Autodesk Inventor part; units mm, degrees
ref_plane "YZ Plane" through (0, 0, 0) normal (1, 0, 0) x (0, 1, 0)
ref_plane "XZ Plane" through (0, 0, 0) normal (0, 1, 0) x (-1, 0, 0)
ref_plane "XY Plane" through (0, 0, 0) normal (0, 0, 1) x (1, 0, 0)
sketch "Sketch1" plane through (0, 0, 0) normal (0, 0, 1) x (1, 0, 0)
  line L0 (10.2242, -22.1045) -> (46.869, -22.1045) construction
  line L1 (46.869, -22.1045) -> (46.869, -51.7203) construction
  line L2 (46.869, -51.7203) -> (10.2242, -51.7203) construction
  line L3 (10.2242, -51.7203) -> (10.2242, -22.1045) construction
  line L4 (29.8676, -31.4438) -> (29.8676, -43.4438) construction
  line L5 (33.8496, -35.029) -> (33.8496, -42.667)
  line L6 (33.8496, -42.667) -> (33.8496, -43.4438)
  line L7 (33.8496, -43.4438) -> (32.8496, -43.4438)
  line L8 (22.8496, -43.4438) -> (22.8496, -42.4438)
  line L9 (22.8496, -31.4438) -> (25.8496, -31.4438)
  line L10 (33.8496, -31.4438) -> (33.8496, -35.019)
  line L11 (28.3496, -31.4438) -> (28.3496, -43.4438) construction
  line L12 (28.3496, -31.4438) -> (25.8496, -31.4438)
  line L13 (25.8496, -31.4438) -> (22.8496, -35.019)
  line L14 (28.3496, -43.4438) -> (23.8496, -43.4438)
  line L15 (23.8496, -43.4438) -> (22.8496, -42.4438)
  line L16 (30.8496, -31.4438) -> (33.8496, -35.019)
  line L17 (32.8496, -43.4438) -> (33.8496, -42.4438)
  line L18 (25.8496, -31.4438) -> (30.8496, -31.4438)
  line L19 (22.8496, -35.019) -> (22.8496, -31.4438)
  line L20 (23.8496, -43.4438) -> (22.8496, -43.4438)
  line L21 (22.8496, -42.4438) -> (22.8496, -35.019)
  line L22 (32.8496, -43.4438) -> (23.8496, -43.4438)
  line L23 (33.8496, -43.4438) -> (33.8496, -43.6998)
  line L24 (33.8496, -42.4438) -> (33.8496, -43.4438)
  line L25 (33.8496, -35.019) -> (33.8496, -42.4438)
  line L26 (30.8496, -31.4438) -> (33.8496, -31.4438)
  circle A0 centre (28.3496, -36.9438) radius 2
  line L27 (26.6175, -35.9438) -> (30.0816, -35.9438)
  line L28 (25.0671, -43.4438) -> (25.3808, -43.8918)
  line L29 (25.0671, -43.4438) -> (25.614, -43.4438) construction
  line L30 (25.3808, -43.8918) -> (25.3808, -45.1736)
  line L31 (25.3808, -45.1736) -> (26.2783, -45.1736)
  line L32 (26.2783, -45.1736) -> (26.2783, -43.9789)
  line L33 (26.2783, -43.9789) -> (26.5414, -43.4438)
  line L34 (27.5656, -43.4438) -> (27.8793, -43.8918)
  line L35 (27.8793, -43.8918) -> (27.8793, -45.1736)
  line L36 (27.8793, -45.1736) -> (28.7769, -45.1736)
  line L37 (28.7769, -45.1736) -> (28.7769, -43.9789)
  line L38 (28.7769, -43.9789) -> (29.04, -43.4438)
  line L39 (31.6321, -43.4438) -> (31.3184, -43.8918)
  line L40 (31.3184, -43.8918) -> (31.3184, -45.1736)
  line L41 (31.3184, -45.1736) -> (30.4209, -45.1736)
  line L42 (30.4209, -45.1736) -> (30.4209, -43.9789)
  line L43 (30.4209, -43.9789) -> (30.1577, -43.4438)
  line L44 (31.6321, -43.4438) -> (31.3184, -43.8918)
  line L45 (31.3184, -43.8918) -> (31.3184, -45.1736)
  line L46 (31.3184, -45.1736) -> (30.4209, -45.1736)
  line L47 (30.4209, -45.1736) -> (30.4209, -43.9789)
  line L48 (30.4209, -43.9789) -> (30.1577, -43.4438)
  line L49 (31.6321, -43.4438) -> (31.3184, -43.8918)
  line L50 (31.3184, -43.8918) -> (31.3184, -45.1736)
  line L51 (31.3184, -45.1736) -> (30.4209, -45.1736)
  line L52 (30.4209, -45.1736) -> (30.4209, -43.9789)
  line L53 (30.4209, -43.9789) -> (30.1577, -43.4438)
  line L54 (28.7769, -30.3247) -> (27.8793, -30.3247)
  line L55 (27.8793, -30.3247) -> (27.8793, -31.4438)
  line L56 (27.8793, -31.4438) -> (28.7769, -31.4438)
  line L57 (28.7769, -31.4438) -> (28.7769, -30.3247)
  point P0 (0, 0)
  dimension "d1" = 12
  dimension "d57" = 11
  dimension "d58" = 2.5
  dimension "d59" = 130
  dimension "d60" = 4.5
  dimension "d61" = 135
  dimension "d66" = 4
  dimension "d69" = 6.5
  dimension "d70" = 3
  dimension "d71" = 55
extrude "Extrusion1" add sketch "Sketch1" along normal blind 2.1 contours L5 L17 L22 L14 L15 L21 L13 L12 L18 L16 L25 | L39 L40 L41 L42 L43 L22 | L18 L12 L55 L54 L57 | L38 L37 L36 L35 L34 L14 L22 | L33 L32 L31 L30 L28 L14
sketch "Sketch2" plane through (0, 0, 2.1) normal (0, 0, 1) x (1, 0, 0)
  line L0 (23.8496, -43.4438) -> (25.0671, -43.4438)
  line L1 (25.0671, -43.4438) -> (32.3568, -43.4438)
  line L2 (32.3568, -43.4438) -> (32.3568, -45.6215)
  line L3 (32.3568, -45.6215) -> (25.0671, -45.6215)
  line L4 (25.0671, -45.6215) -> (25.0671, -43.4438)
  line L5 (27.8793, -30.3247) -> (27.8793, -31.4438)
  line L6 (28.7769, -31.4438) -> (28.7769, -30.3247)
  line L7 (27.8793, -31.4438) -> (28.7769, -31.4438)
  line L8 (28.7769, -31.4438) -> (28.7769, -30.3247)
  line L9 (28.7769, -30.3247) -> (27.8793, -30.3247)
  line L10 (27.8793, -30.3247) -> (27.8793, -31.4438)
  point P0 (0, 0)
extrude "Extrusion2" cut sketch "Sketch2" against normal blind 1.5
properties part number "mainbody"
The listing builds one solid part. Answer for the finished solid, in the listing's coordinates (mm). A direction names the side the tool comes from. Coordinates: 2 decimals unless noted, no trailing zeros. Write each loop counter-clockwise with the first axis right and the second up, starting at its lowest first coordinate (ties: lowest second). Pieces come first, ordered by that corner, then holes. Notation, with made-up numbers: M 31.25,62 L 54.25,62 A12 cw 54.25,85 Z; hole C 70.5,61 d8. An arc over 180 degrees is marked long. Put each result on its own line as item: value. Start each with the question number.
1. A cutting plane is placed at D-D on x = 32.5. Write down the section's boundary in (y, z).
2. A cutting plane is placed at B-B on x = 29.25. Write down the section's boundary in (y, z), then the cut area to 3 significant figures.
3. Flat-ended cylindrical pins translate along their axes: P1, Ø0.5, axis at y = -31, z = 0, coming from the -X side; P2, Ø0.6, axis at x = 29, z = 1.5, coming from the +Y side; P3, Ø0.7, axis at x = 28, y = -44, coming from the +Z side. Find the tip coordinate at first contact, or state that the pin passes through.
4. A cutting plane is placed at C-C on z = 1.35. Write down the section's boundary in (x, y).
5. Which of the six approach directions +Z, -Z, +X, -X, +Y, -Y give full straight-line access (tool end or side, diameter ignored) to faces 1 (the flat face through (31, -44, 0.6)), 2 (the flat face through (28.3, -30.9, 0.6)), 3 (the flat face through (33.85, -39, 1)), 4 (the flat face through (28, -43.444, 1))?
6. For a pull along X with two mould halves and no side action, classify faces 5 (the cylindrical face through (29.27, -35.17, 1.04)), 6 (the flat face through (33.343, -42.951, 1.035)), 7 (the flat face through (22.85, -39, 1)), 8 (the flat face through (28, -31.444, 1)) as pulls with the +X half, pulls with the -X half, needs draft (parallel to the pull), parting line crosses it, or undercut.
7. A cutting plane is placed at A-A on y = -38. Write down the section's boundary in (x, z).
8. Consider line 1 (Y direction, x = 26, z = 1.75); line 2 (X direction, y = -35.25, z = 2); line 3 (Y direction, x = 28.5, z = 0.85). Determine where each line is inside the solid, lowest interval first. Write a range as from..to.
Resolved:
1. outline: M -43.44,0 L -33.41,0 L -33.41,2.1 L -43.44,2.1 Z
2. outline: M -43.44,0 L -38.73,0 L -38.73,2.1 L -43.44,2.1 Z; M -35.16,0 L -31.44,0 L -31.44,2.1 L -35.16,2.1 Z
2. area: 17.7 mm2
3. P1: stops at x = 27.88
3. P2: stops at y = -31.44
3. P3: stops at z = 0.6
4. outline: M 22.85,-42.44 L 23.85,-43.44 L 32.85,-43.44 L 33.85,-42.44 L 33.85,-35.02 L 30.85,-31.44 L 25.85,-31.44 L 22.85,-35.02 Z; hole C 28.35,-36.94 d4
5. face 1: +Z, +X, -X, -Y
5. face 2: +Z, +X, -X, +Y
5. face 3: +Z, -Z, +X, +Y, -Y
5. face 4: +Z, -Y
6. face 5: undercut
6. face 6: pulls with the +X half
6. face 7: pulls with the -X half
6. face 8: needs draft
7. outline: M 22.85,0 L 26.65,0 L 26.65,2.1 L 22.85,2.1 Z; M 30.05,0 L 33.85,0 L 33.85,2.1 L 30.05,2.1 Z
8. line 1: y = -43.44..-31.44
8. line 2: x = 22.85..27.29, 29.41..33.85
8. line 3: y = -43.44..-38.94, -34.95..-31.44
